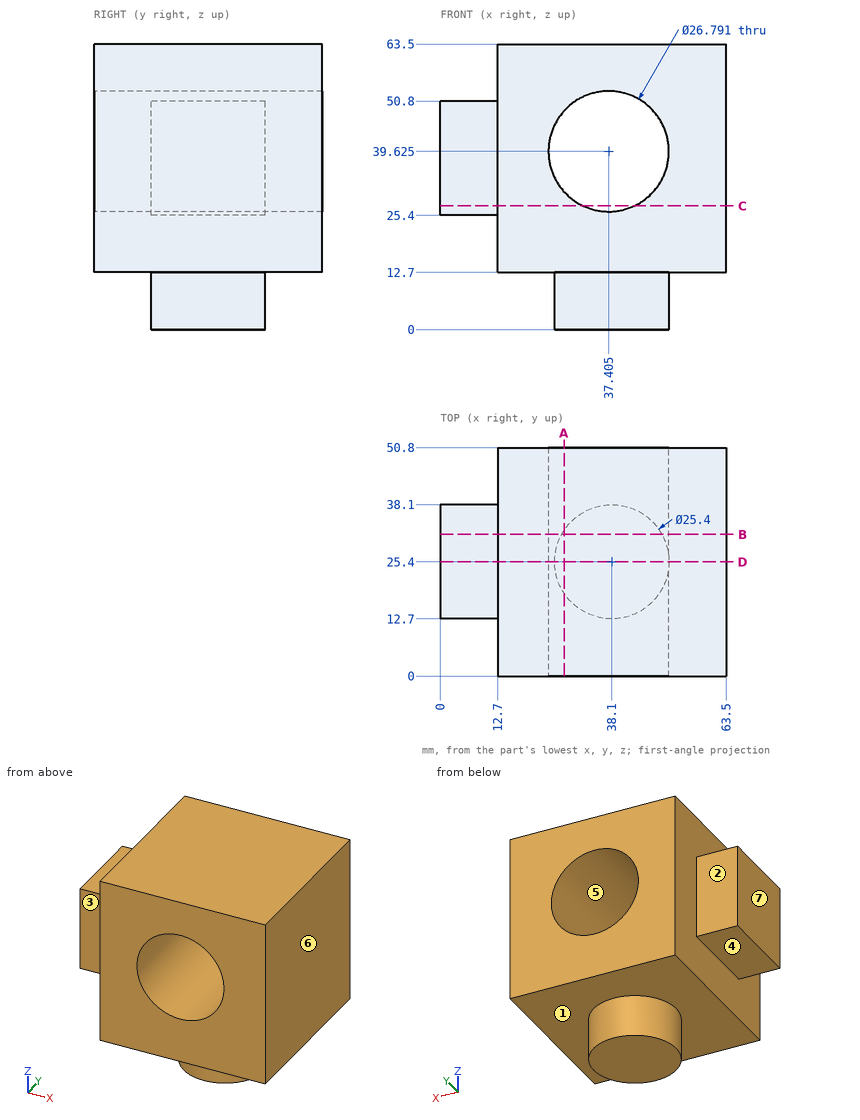
Verification items for this drawing (mm, ordinates from the low corner). A direction names the side the tool comes from. Give positions to 0.01 mm unless a question says otherwise; leave off trailing zeros. Loops run counter-clockwise (first coordinate to the right, second up) from the corner with the lowest first, then second, coordinate; pieces in that order, holes last. Notation, with made-up numbers: M 21.5,4.25 L 72.5,4.25 A9 cw 72.5,11.25 Z; hole C 37,62.25 d9. An arc over 180 degrees is marked long. Answer as a JSON object with one key per item and string values. Group by question number.
Item 1: Sectioned sample at B-B on y = 31.5. Record the boundary of the cut face in (x, z) (1 decimal).
Item 2: Sectioned sample at D-D on y = 25.4. Record the boundary of the cut face in (x, z) (1 decimal).
Item 3: Mould release check, pull along X, two halves, no side actions. Record for the marked faces 5, 6 and 7: pulls with the +X half, pulls with the -X half, needs draft (parallel to the pull), parting line crosses it, or undercut.
Item 4: Access from +Z, -Z, +X, -X, +Y, -Y to the whole of each face (thin tool, end or side, straight path). Record for the marked faces 1, 2, 3 and 4.
Item 5: Sectioned sample at C-C on z = 27.5. Record the boundary of the cut face in (x, y), plus the area to 3 significant figures.
Item 6: Material ranges on L1, parallel to Z at x = 21.5, y = 47; L2, parallel to X at y = 26.5, z = 28.5 (1 decimal), recorded low to high.
Item 7: Gauge pin test, flat ends, axial feed: pin 1 (10 mm diameter, centred on x = 6, z = 39.5, fed in from -Y); pin 2 (6 mm diameter, centred on y = 44, z = 23.5, fed in from -X); pin 3 (10 mm diameter, centred on x = 7, y = 24.5, fed in from -Z); pin 4 (24 mm diameter, centred on x = 37.4, z = 39.62, fed in from +Y). Record the tip position at first contact, or that the pin passes through.
Item 8: Sectioned sample at A-A on x = 27.5. Record the boundary of the cut face in (y, z) (1 decimal), plus the area to 3 significant figures.
Findings below:
{
 "1": {"outline": "M 0,25.4 L 12.7,25.4 L 12.7,12.7 L 27,12.7 L 27,0 L 49.2,0 L 49.2,12.7 L 63.5,12.7 L 63.5,63.5 L 12.7,63.5 L 12.7,50.8 L 0,50.8 Z; hole C 37.4,39.6 d26.8"},
 "2": {"outline": "M 0,25.4 L 12.7,25.4 L 12.7,12.7 L 25.4,12.7 L 25.4,0 L 50.8,0 L 50.8,12.7 L 63.5,12.7 L 63.5,63.5 L 12.7,63.5 L 12.7,50.8 L 0,50.8 Z; hole C 37.4,39.6 d26.8"},
 "3": {"face 5": "undercut", "face 6": "pulls with the +X half", "face 7": "pulls with the -X half"},
 "4": {"face 1": "-Z", "face 2": "+Z, -Z, -X, +Y", "face 3": "+Z, -Z, -X, -Y", "face 4": "-Z, -X, +Y, -Y"},
 "5": {"outline": "M 0,12.7 L 12.7,12.7 L 12.7,0 L 31.71,0 L 31.71,50.8 L 12.7,50.8 L 12.7,38.1 L 0,38.1 Z; M 43.1,0 L 63.5,0 L 63.5,50.8 L 43.1,50.8 Z", "area": "2,320 mm2"},
 "6": {"L1": "12.7 to 63.5", "L2": "0 to 29.9, 44.9 to 63.5"},
 "7": {"pin 1": "y = 12.7", "pin 2": "x = 12.7", "pin 3": "z = 25.4", "pin 4": "through"},
 "8": {"outline": "M 0,12.7 L 18.4,12.7 L 18.4,0 L 32.4,0 L 32.4,12.7 L 50.8,12.7 L 50.8,30.6 L 0,30.6 Z; M 0,48.6 L 50.8,48.6 L 50.8,63.5 L 0,63.5 Z", "area": "1,840 mm2"}
}
